Design review of the part built by this model. Coordinates are the model's own, in mm. A direction names the side the tool comes from. Coordinates: 2 decimals unless noted, no trailing zeros. Loops run counter-clockwise (first coordinate to the right, second up) from the corner with the lowest first, then second, coordinate; pieces in that order, holes last.
Q1. Add section A-A on z = 2.5. Give the boundary of the cut face in (x, y).
Q2. Machinability: for faces 1 (the face through (17, -16, 0)), 2 (the face through (6, -28, 4.05)), 3 (the face through (5, -13, 5)), which of the approach directions +Z, -Z, +X, -X, +Y, -Y give a long, thin tool a straight path to every point of the face, cutting with its end or side? Answer none if there is none.
Q3. Add section D-D on x = 0. Give the boundary of the cut face in (y, z).
Q4. Wall thickness on probe 1 along X at (y, z) = (-24, 21); probe 2 along X at (y, z) = (-2, 9.5); probe 3 along Y at (x, z) = (-3.5, 13): over which ranges is each line inside the solid? List them lowest first.
Q5. For P1, Ø4, axis at y = -24, z = 14, coming from the +X side; P2, Ø1.2, axis at x = 5.5, y = -27.5, coming from the +Z side; P3, Ø10.5, axis at y = -9, z = 5.5, coming from the -X side, all flat-tipped, find the tip position at first contact; note any pin that passes through.
Q6. Add section B-B on y = -13. Give the boundary of the cut face in (x, z) (3 decimals), and give its area (3 significant figures).
Q7. Add section C-C on z = 21. Give the boundary of the cut face in (x, y), and give its area (3 significant figures).
Q8. Draft analysis for pull direction X (two halves, no side actions). For faces 4 (the face through (0, -11, 9.678)), 5 (the face through (19.87, -16.27, 13.31)), 6 (the face through (0, 0, 11)), state which applies: released by +X, released by -X, zero draft, split by the parting line, or undercut.
```python
from build123d import *

# Parameters (mm, degrees)
F1_DEPTH = 33
F2_W     = 10
F2_H     = 9.678203
F3_DEPTH = 33
F4_W     = 13
F4_H     = 22.949062
F5_DEPTH = 11


with BuildPart() as f1:
    # F0 (on Front) → F1 (new body)
    with BuildSketch(Plane.XZ):
        Polygon((10.25, 26.999062), (-10.25, 26.999062), (-29.225, 0), (29.225, 0), align=None)
    extrude(amount=F1_DEPTH)

    # F2 (on face) → F3 (cut)
    with BuildSketch(Plane.XZ.offset(33)):
        with Locations((0, 4.839101)):
            Rectangle(F2_W, F2_H)
    extrude(amount=-F3_DEPTH, mode=Mode.SUBTRACT)

    # F4 (on face) → F5 (cut)
    with BuildSketch(Plane.XZ.offset(33)):
        with Locations((0, 15.524531)):
            Rectangle(F4_W, F4_H)
    extrude(amount=-F5_DEPTH, mode=Mode.SUBTRACT)


solid = f1.part
```
Entries:
1. outline: (-27.47, -33) - (-5, -33) - (-5, 0) - (-27.47, 0) - close; (5, -33) - (27.47, -33) - (27.47, 0) - (5, 0) - close
2. face 1: -Z, +X, -X, +Y, -Y
2. face 2: +Z, -Y
2. face 3: -Z, +Y, -Y
3. outline: (-22, 9.68) - (0, 9.68) - (0, 27) - (-22, 27) - close
4. probe 1: x = -14.47 to -6.5, 6.5 to 14.47
4. probe 2: x = -22.55 to -5, 5 to 22.55
4. probe 3: y = -22 to 0
5. P1: stops at x = 20.79
5. P2: stops at z = 4.05
5. P3: stops at x = -29.05
6. outline: (-29.225, 0) - (-5, 0) - (-5, 9.678) - (5, 9.678) - (5, 0) - (29.225, 0) - (10.25, 26.999) - (-10.25, 26.999) - close
6. area: 969 mm2
7. outline: (-14.47, -33) - (-6.5, -33) - (-6.5, -22) - (6.5, -22) - (6.5, -33) - (14.47, -33) - (14.47, 0) - (-14.47, 0) - close
7. area: 812 mm2
8. face 4: undercut
8. face 5: released by +X
8. face 6: zero draft
